Geometry check sheet. Reference: drawing and pictorial views, mm from the part's lowest x, y, z. A direction names the side the tool comes from. Give positions to 0.01 mm unless a question says otherwise; leave off trailing zeros. Order: outer loops, then holes, each group sorted by start corner. A loop starts at its lowest first (then second) coordinate and runs counter-clockwise, first axis right, second up.
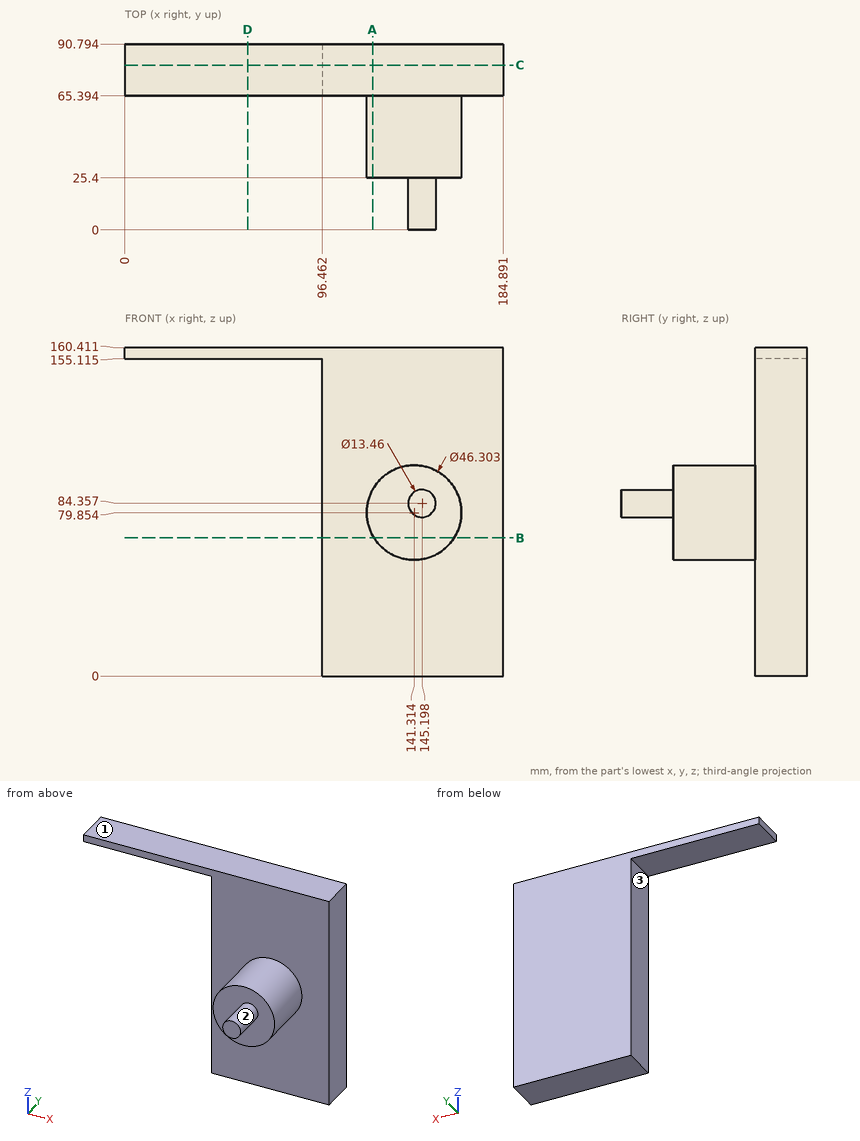
(1) Sectioned sample at D-D (x = 60). Enter the section's corners in (y, z) (1 decimal).
(2) Tool access check on the marked faces 1, 2 and 3. Record the directions out of +Z, -Z, +X, -X, +Y, -Y that give a thin tool (end or side, any length) a straight path to the whole face; none if there is none.
(3) Go/stop test with flat-tipped pins: P1, Ø10, axis at y = 58, z = 69, coming from the -X side (1 decimal); P2, Ø10, axis at y = 47.5, z = 55.5, coming from the +X side; P3, Ø20.5, axis at y = 76.5, z = 65, coming from the -X side. Record where each tip stops, or that it passes through.
(4) Sectioned sample at C-C (y = 80.5). Enter the section's corners in (x, z) (1 decimal).
(5) Sectioned sample at A-A (x = 121). Enter the section's corners in (y, z) (1 decimal).
(6) Thickness scan on L1, parallel to X at y = 80, z = 140; L2, parallel to Z at x = 72, y = 75.5 (1 decimal); L3, parallel to Y at x = 128.5, z = 125.5 (1 decimal). Record the ranges inside material, lowest first.
(7) Sectioned sample at B-B (z = 67.5). Enter the section's corners in (x, y) (1 decimal), plus the area to 3 significant figures.
Values follow:
1. outline: (65.4, 155.1) - (90.8, 155.1) - (90.8, 160.4) - (65.4, 160.4) - close
2. face 1: +Z, +X, -X, +Y, -Y
2. face 2: -Y
2. face 3: -Z, -X, +Y, -Y
3. P1: stops at x = 118.9
3. P2: stops at x = 154.02
3. P3: stops at x = 96.46
4. outline: (0, 155.1) - (96.5, 155.1) - (96.5, 0) - (184.9, 0) - (184.9, 160.4) - (0, 160.4) - close
5. outline: (25.4, 68.7) - (65.4, 68.7) - (65.4, 0) - (90.8, 0) - (90.8, 160.4) - (65.4, 160.4) - (65.4, 91) - (25.4, 91) - close
6. L1: x = 96.46 to 184.89
6. L2: z = 155.1 to 160.4
6. L3: y = 65.4 to 90.8
7. outline: (96.5, 65.4) - (121.7, 65.4) - (121.7, 25.4) - (160.9, 25.4) - (160.9, 65.4) - (184.9, 65.4) - (184.9, 90.8) - (96.5, 90.8) - close
7. area: 3,810 mm2
